Source: CAD feature listing. Evaluate the final solid. Frame: model axes, mm. A direction names the side the tool comes from. Give positions to 0.01 mm unless a question says otherwise; leave off trailing zeros. Order: outer loops, then holes, each group sorted by start corner. A loop starts at its lowest first (then second) coordinate and runs counter-clockwise, first axis right, second up. Notation, with made-up numbers: (22.25, 1.5) - (70.25, 1.5) arc R36 ccw to (70.25, 39.5) - close; hole circle Ø9 at (-1.5, 58.25). An arc over 180 degrees is marked (long way). Write each question's results on one line, items separated by ' | '. Start each with the question number.
Item 1: Set-up query: faces 4 (the cylindrical face through (45.773, 12.789, 35.474)), 5 (the flat face through (55, 19.05, 25)). Return all of +Z, -Z, +X, -X, +Y, -Y with unobstructed straight access to the full face (end or side cutting, diameter ignored); none if empty.
Item 2: Line query: line 1 along Z through (x, y) = (44.45, 2.5); line 2 along X through (y, z) = (6, 8); line 3 along X through (y, z) = (4, 6.5). Output: solid intervals per line, ascending.
Item 3: Section A-A on x = 44.45. Output: boundary loops of the cut face in (y, z).
Item 4: Section C-C on z = 25.4. Output: boundary loops of the cut face in (x, y), and give its area (3 significant figures).
Item 5: Section D-D on z = 43. Output: boundary loops of the cut face in (x, y).
Item 6: Mould query, pull axis X, two halves, no side actions, for faces 1 (the flat face through (45, 6.35, 21)), 2 (the flat face through (88.9, 9, 25)), 3 (the flat face through (44, 12, 50.8)). Classes: released by +X, released by -X, zero draft, split by the parting line, or undercut.
Item 7: Section B-B on y = 2. State how many separate pieces and enclosed holes the cut face has, and give its area (3 significant figures).
Item 8: Contact query for flat-ended pins moving along their axis: pin 1 Ø2 at (x, z) = (10.5, 44) entering from -Y; pin 2 Ø22.5 at (x, z) = (45.5, 28.5) entering from +Y. Output: stop coordinate, or through.
```python
from build123d import *

# Parameters (mm, degrees)
F1_DEPTH = 50.8
F2_R     = 10.16
F3_DEPTH = 12.7
F4_R     = 3.4925
F5_DEPTH = 6.351


with BuildPart() as f1:
    # F0 (on Top) → F1 (new body)
    with BuildSketch(Plane.XY):
        with BuildLine():
            Line((0, 19.05), (0, 0))
            Line((0, 0), (6.35, 0))
            ThreePointArc((6.35, 0), (19.05, 12.7), (31.75, 0))
            Line((31.75, 0), (57.15, 0))
            ThreePointArc((57.15, 0), (69.85, 12.7), (82.55, 0))
            Line((82.55, 0), (88.9, 0))
            Line((88.9, 0), (88.9, 19.05))
            Line((88.9, 19.05), (0, 19.05))
        make_face()
    extrude(amount=F1_DEPTH)

    # F2 (on face) → F3 (cut)
    with BuildSketch(Plane(origin=(0, 19.05, 0), x_dir=(-1, 0, 0), z_dir=(0, 1, 0))):
        with Locations((-44.45, 25.4)):
            Circle(F2_R)
    extrude(amount=-F3_DEPTH, mode=Mode.SUBTRACT)

    # F4 (on face) → F5 (cut, through all)
    with BuildSketch(Plane(origin=(0, 6.35, 0), x_dir=(-1, 0, 0), z_dir=(0, 1, 0))):
        with Locations((-44.45, 25.4)):
            Circle(F4_R)
    extrude(amount=-F5_DEPTH, mode=Mode.SUBTRACT)


solid = f1.part
```
Evaluation:
1) face 4: +Y | face 5: +Z, -Z, +X, -X, +Y
2) line 1: z = 0 to 21.91, 28.89 to 50.8 | line 2: x = 0 to 7.86, 30.24 to 58.66, 81.04 to 88.9 | line 3: x = 0 to 7, 31.1 to 57.8, 81.9 to 88.9
3) outline: (0, 0) - (19.05, 0) - (19.05, 15.24) - (6.35, 15.24) - (6.35, 21.91) - (0, 21.91) - close; (0, 28.89) - (6.35, 28.89) - (6.35, 35.56) - (19.05, 35.56) - (19.05, 50.8) - (0, 50.8) - close
4) outline: (0, 0) - (6.35, 0) arc R12.7 cw to (31.75, 0) - (40.96, 0) - (40.96, 6.35) - (34.29, 6.35) - (34.29, 19.05) - (0, 19.05) - close; (47.94, 0) - (57.15, 0) arc R12.7 cw to (82.55, 0) - (88.9, 0) - (88.9, 19.05) - (54.61, 19.05) - (54.61, 6.35) - (47.94, 6.35) - close | area: 884 mm^2
5) outline: (0, 0) - (6.35, 0) arc R12.7 cw to (31.75, 0) - (57.15, 0) arc R12.7 cw to (82.55, 0) - (88.9, 0) - (88.9, 19.05) - (0, 19.05) - close
6) face 1: undercut | face 2: released by +X | face 3: zero draft
7) separate pieces: 3 | enclosed holes: 1 | area: 1,930 mm^2
8) pin 1: stops at y = 8.37 | pin 2: stops at y = 19.05
